Can you work these out from the model? Positions are in its coordinate system, mm. Face numbers are marked on the shaded views. A direction names the side the tool comes from. Coordinates: 2 decimals unless noted, no trailing zeros. Order: outer loops, then holes, each group sorted by start corner. A loop starts at its lowest first (then second) coordinate and runs counter-clockwise, first axis right, second up. Notation, with made-up numbers: (16.25, -26.75) -> (54.25, -26.75) arc R28 cw to (54.25, 3.25) -> close; hole circle Ø6 at (-30.5, 8). An arc over 180 degrees is marked (long way). Return JSON: item names as keys, results as strings. Group by question number.
1) If we section it at C-C, the plane z = 1: Please give me the cut outline in (x, y), then the cut area to 3 significant figures.
2) If I drill on probe 1 along Y at (x, z) = (7, 7); probe 2 along Y at (x, z) = (25.5, 28); probe 3 along X at (y, z) = (5, 21), over which ranges is the centre line in solid material (lowest first)? Write a range as from..to.
3) If we section it at B-B, the plane x = 7: Please give me the cut outline in (y, z).
4) Thinking about a two-plate mould opening in Y: for the marked faces 4, 5 and 6, which applies, +Y half, -Y half, draft (parallel to the pull), parting line (faces both ways), or undercut?
5) For pin 1 (8 mm diameter, centred on y = 51, z = 3.5, fed in from +X); pin 2 (12 mm diameter, centred on x = 22.5, z = -5.5, fed in from -Y); pin 3 (1.5 mm diameter, centred on x = 45.5, z = 18, fed in from +Y); pin 4 (6 mm diameter, centred on x = 13.5, y = 54, fed in from +Z), each with a flat end and sliding along its axis, tell me the tip position at first contact or that it passes through.
6) If we section it at A-A, the plane y = 58: Please give me the cut outline in (x, z).
7) For the marked faces 1, 2 and 3, which set-ups out of +Z, -Z, +X, -X, +Y, -Y let a thin tool reach every point of the face, with its end or its side?
8) If we section it at D-D, the plane x = 56.5: Please give me the cut outline in (y, z), then the cut area to 3 significant figures.
Autodesk Inventor part; units mm, degrees
ref_plane "YZ Plane" through (0, 0, 0) normal (1, 0, 0) x (0, 1, 0)
ref_plane "XZ Plane" through (0, 0, 0) normal (0, 1, 0) x (-1, 0, 0)
ref_plane "XY Plane" through (0, 0, 0) normal (0, 0, 1) x (1, 0, 0)
sketch "Sketch1" plane through (0, 0, 0) normal (0, 0, 1) x (1, 0, 0)
  line L0 (0, 0) -> (0, 65)
  line L1 (0, 65) -> (60, 65)
  line L2 (60, 0) -> (0, 0)
  line L3 (60, 13.6397) -> (65, 11.8199)
  line L4 (65, 11.8199) -> (65, 21.8199)
  line L5 (65, 21.8199) -> (60, 20)
  line L6 (60, 13.6397) -> (60, 0)
  line L7 (60, 40) -> (65, 41.8199)
  line L8 (65, 41.8199) -> (65, 31.8199)
  line L9 (65, 31.8199) -> (60, 33.6397)
  line L10 (60, 65) -> (60, 40)
  line L11 (60, 33.6397) -> (60, 20)
  circle A0 centre (7, 58) radius 5
  dimension "d0" = 65
  dimension "d1" = 60
  dimension "d2" = 10
  dimension "d6" = 6.3603
  dimension "d7" = 5
  dimension "d8" = 20
  dimension "d10" = 70
  dimension "d11" = 13.6397
  dimension "d12" = 10
  dimension "d13" = 70
  dimension "d14" = 70
  dimension "d15" = 70
  dimension "d16" = 5
  dimension "d17" = 40
  dimension "d18" = 10
  dimension "d19" = 7
  dimension "d20" = 7
extrude "Extrusion1" add sketch "Sketch1" along normal blind 10
sketch "Sketch2" plane through (0, 0, 0) normal (0, 0, -1) x (-1, 0, 0)
  line L0 (0, 65) -> (0, 0)
  line L1 (0, 0) -> (0, 10)
  line L2 (0, 10) -> (-60, 10)
  line L3 (-60, 0) -> (-60, 13.6397)
  line L4 (-60, 0) -> (0, 0)
  dimension "d23" = 10
sketch "Sketch3" plane through (0, 0, 0) normal (0, 0, -1) x (-1, 0, 0)
  point P0 (0, 0)
extrude "Extrusion2" add sketch "Sketch2" along normal blind 20
fillet "Fillet1" radius 3 1 edges at (30, 10, 0)
sketch "Sketch4" plane through (0, 0, 10) normal (0, 0, 1) x (1, 0, 0)
  line L0 (0, 0) -> (0, 10)
  line L1 (60, 10) -> (60, 13)
  line L2 (0, 10) -> (60, 10)
  line L3 (60, 10) -> (60, 0)
  line L4 (0, 0) -> (60, 0)
  line L5 (60, 0) -> (0, 0)
  line L6 (0, 0) -> (0, 10)
extrude "Extrusion3" add sketch "Sketch4" along normal blind 20
properties part number "SpoolWinderDriveBase"
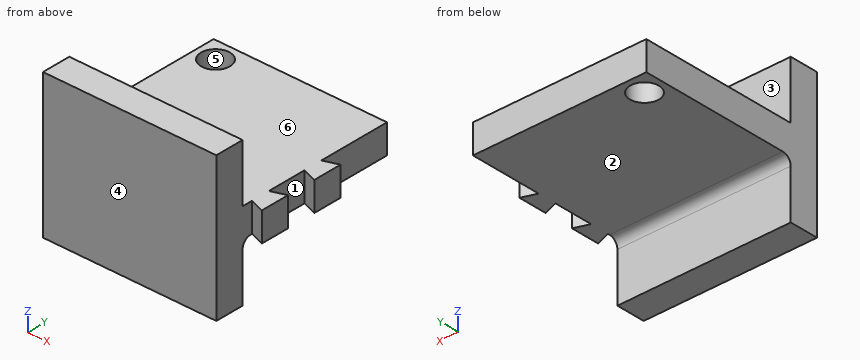
Result sheet:
{
 "1": {"outline": "(0, 0) -> (60, 0) -> (60, 13.64) -> (65, 11.82) -> (65, 21.82) -> (60, 20) -> (60, 33.64) -> (65, 31.82) -> (65, 41.82) -> (60, 40) -> (60, 65) -> (0, 65) -> close; hole circle Ø10 at (7, 58)", "area": "3,900 mm2"},
 "2": {"probe 1": "y = 0..53, 63..65", "probe 2": "y = 0..10", "probe 3": "x = 0..60"},
 "3": {"outline": "(0, -20) -> (10, -20) -> (10, -3) arc R3 cw to (13, 0) -> (53, 0) -> (53, 10) -> (10, 10) -> (10, 30) -> (0, 30) -> close; (63, 0) -> (65, 0) -> (65, 10) -> (63, 10) -> close"},
 "4": {"face 4": "-Y half", "face 5": "undercut", "face 6": "draft"},
 "5": {"pin 1": "stops at x = 60", "pin 2": "stops at y = 0", "pin 3": "stops at y = 10", "pin 4": "stops at z = 10"},
 "6": {"outline": "(0, 0) -> (2, 0) -> (2, 10) -> (0, 10) -> close; (12, 0) -> (60, 0) -> (60, 10) -> (12, 10) -> close"},
 "7": {"face 1": "+Z, -Z", "face 2": "-Z, +X, -X, +Y", "face 3": "+Z, +X, -X, +Y"},
 "8": {"outline": "(0, -20) -> (10, -20) -> (10, -3) arc R3 cw to (13, 0) -> (65, 0) -> (65, 10) -> (10, 10) -> (10, 30) -> (0, 30) -> close", "area": "1,050 mm2"}
}
